Work out the finished part from the listing and answer in its coordinate system (mm). Round coordinates to 2 decimals unless told otherwise and drop trailing zeros. Order: outer loops, then holes, each group sorted by start corner. A loop starts at its lowest first (then second) coordinate and runs counter-clockwise, first axis right, second up. Notation, with made-up numbers: M 52,-37 L 107,-37 A15 ccw 107,-9 Z; hole C -22.75,67.5 d4. An arc over 180 degrees is marked long. Return JSON: item names as keys, results as strings.
from build123d import *

# Parameters (mm, degrees)
BOSS_EXTRUDE1_DEPTH = 7
SKETCH2_R           = 7
BOSS_EXTRUDE3_DEPTH = 7
SKETCH3_R           = 7
CUT_EXTRUDE1_DEPTH  = 7


with BuildPart() as part:
    # Sketch1 → Boss-Extrude1 (new body)
    with BuildSketch(Plane.XY):
        with BuildLine():
            Line((-75, 15), (75, 15))
            ThreePointArc((75, 15), (90, 0), (75, -15))
            Line((75, -15), (-75, -15))
            ThreePointArc((-75, -15), (-90, 0), (-75, 15))
        make_face()
    extrude(amount=BOSS_EXTRUDE1_DEPTH)

    # Sketch2 → Boss-Extrude3 (add)
    with BuildSketch(Plane.XY):
        with Locations((75, 0)):
            Circle(SKETCH2_R)
    extrude(amount=-BOSS_EXTRUDE3_DEPTH)

    # Sketch3 → Cut-Extrude1 (cut)
    with BuildSketch(Plane(origin=(0, 0, 0), x_dir=(-1, 0, 0), z_dir=(0, 0, -1))):
        with Locations((75, 0)):
            Circle(SKETCH3_R)
    extrude(amount=-CUT_EXTRUDE1_DEPTH, mode=Mode.SUBTRACT)


solid = part.part
Item 1: Consider line 1 along Y through (x, z) = (-75, 3); line 2 along Z through (x, y) = (23, -2); line 3 along X through (y, z) = (2, 4.75). Determine where each line is inside the solid, lowest interval first. Write a range as [from, to].
Output:
{"line 1": "y = [-15, -7], [7, 15]", "line 2": "z = [0, 7]", "line 3": "x = [-89.87, -81.71], [-68.29, 89.87]"}
Item 2: Each of these flat-tipped pins is pushed along its axis until it touches: pin 1 (8 mm diameter, centred on x = 31, y = 8.5, fed in from -Z); pin 2 (1 mm diameter, centred on y = 1.5, z = 5, fed in from +X); pin 3 (3 mm diameter, centred on y = 6.5, z = -4.5, fed in from +X). Where does it stop, or does it pass through?
Output:
{"pin 1": "stops at z = 0", "pin 2": "stops at x = 89.97", "pin 3": "stops at x = 79.9"}
Item 3: Find section D-D (x = -56). Determine the outline of the cut face in (y, z), plus the area to 3 significant figures.
Output:
{"outline": "M -15,0 L 15,0 L 15,7 L -15,7 Z", "area": "210 mm^2"}
Item 4: The mould has two halves that part along Y. Classify faces 1 (the flat face through (1, 0, 7)), 2 (the cylindrical face through (-68, 0, 3)), 3 (the cylindrical face through (68, 0, -3)): pulls with the +Y half, pulls with the -Y half, needs draft (parallel to the pull), parting line crosses it, or undercut.
Output:
{"face 1": "needs draft", "face 2": "undercut", "face 3": "parting line crosses it"}
Item 5: Find section C-C (z = -4.75). Determine the outline of the cut face in (x, y).
Output:
{"outline": "C 75,0 d14"}
Item 6: Find section B-B (z = 2.5). Determine the outline of the cut face in (x, y), plus the area to 3 significant figures.
Output:
{"outline": "M -75,-15 L 75,-15 A15 ccw 75,15 L -75,15 A15 ccw Z; hole C -75,0 d14", "area": "5,050 mm^2"}
Item 7: Find section A-A (y = 0). Determine the outline of the cut face in (x, z), plus the area to 3 significant figures.
Output:
{"outline": "M -90,0 L -82,0 L -82,7 L -90,7 Z; M -68,0 L 68,0 L 68,-7 L 82,-7 L 82,0 L 90,0 L 90,7 L -68,7 Z", "area": "1,260 mm^2"}
